from build123d import *

# Parameters (mm, degrees)
SKETCH1_W           = 80
SKETCH1_H           = 68
BOSS_EXTRUDE1_DEPTH = 45
CUT_EXTRUDE1_START  = 45
SKETCH2_W           = 76
SKETCH2_H           = 64
CUT_EXTRUDE1_DEPTH  = 33
SKETCH6_R           = 10.5
CUT_EXTRUDE10_DEPTH = 5
SKETCH7_W           = 30
SKETCH7_H           = 30
SKETCH7_W_2         = 26
SKETCH7_H_2         = 26
CUT_EXTRUDE11_DEPTH = 2
SKETCH8_R           = 1.5
CUT_EXTRUDE12_DEPTH = 3
SKETCH5_R           = 5.95
CUT_EXTRUDE14_DEPTH = 46
FILLET1_R           = 0.5
CUT_EXTRUDE15_START = 12
SKETCH12_R          = 24
CUT_EXTRUDE15_DEPTH = 5.5
BOSS_EXTRUDE5_START = -34
SKETCH13_W          = 80
SKETCH13_H          = 45
BOSS_EXTRUDE5_DEPTH = 16
CUT_EXTRUDE16_START = 45
SKETCH15_W          = 25
SKETCH15_H          = 16
CUT_EXTRUDE16_DEPTH = 33
SKETCH16_R          = 5.95
CUT_EXTRUDE17_DEPTH = 10
CUT_EXTRUDE18_START = 40
SKETCH17_R          = 5.6
CUT_EXTRUDE18_DEPTH = 50
CUT_EXTRUDE19_START = 40
SKETCH20_R          = 1
CUT_EXTRUDE19_DEPTH = 53
FILLET3_R           = 2
FILLET4_R           = 2
CUT_EXTRUDE20_START = 45
SKETCH21_W          = 51
SKETCH21_H          = 2
CUT_EXTRUDE20_DEPTH = 2
CUT_EXTRUDE22_START = 45
SKETCH22_W          = 2
SKETCH22_H          = 14
CUT_EXTRUDE22_DEPTH = 2
CUT_EXTRUDE23_START = -40
CUT_EXTRUDE23_DEPTH = 2


with BuildPart() as part:
    # Sketch1 → Boss-Extrude1 (new body)
    with BuildSketch(Plane(origin=(0, 0, 0), x_dir=(1, 0, 0), z_dir=(0, 1, 0))):
        Rectangle(SKETCH1_W, SKETCH1_H)
    extrude(amount=BOSS_EXTRUDE1_DEPTH)

    # Sketch2 → Cut-Extrude1 (cut)
    with BuildSketch(Plane(origin=(0, 0, 0), x_dir=(1, 0, 0), z_dir=(0, 1, 0)).offset(CUT_EXTRUDE1_START)):
        Rectangle(SKETCH2_W, SKETCH2_H)
    extrude(amount=-CUT_EXTRUDE1_DEPTH, mode=Mode.SUBTRACT)

    # Sketch6 → Cut-Extrude10 (cut)
    with BuildSketch(Plane.XZ):
        Circle(SKETCH6_R)
    extrude(amount=-CUT_EXTRUDE10_DEPTH, mode=Mode.SUBTRACT)

    # Sketch7 → Cut-Extrude11 (cut)
    with BuildSketch(Plane(origin=(0, 0, 0), x_dir=(-1, 0, 0), z_dir=(0, -1, 0))):
        Rectangle(SKETCH7_W, SKETCH7_H)
        Rectangle(SKETCH7_W_2, SKETCH7_H_2, mode=Mode.SUBTRACT)
    extrude(amount=-CUT_EXTRUDE11_DEPTH, mode=Mode.SUBTRACT)

    # Sketch8 → Cut-Extrude12 (cut, through all)
    with BuildSketch(Plane.ZY.offset(-38)):
        with Locations((29, 17)):
            Circle(SKETCH8_R)
    extrude(amount=-CUT_EXTRUDE12_DEPTH, mode=Mode.SUBTRACT)

    # Sketch5 → Cut-Extrude14 (cut, through all)
    with BuildSketch(Plane(origin=(0, 0, 0), x_dir=(1, 0, 0), z_dir=(0, 1, 0))):
        Circle(SKETCH5_R)
    extrude(amount=CUT_EXTRUDE14_DEPTH, mode=Mode.SUBTRACT)

    # Fillet1
    fillet1_edges = [part.edges().sort_by_distance(p)[0] for p in [
        (15, 0, 0),
        (0, 0, 15),
        (-15, 0, 0),
        (0, 0, -15),
        (13, 0, 0),
        (0, 0, -13),
        (-13, 0, 0),
        (0, 0, 13),
    ]]
    fillet(fillet1_edges, radius=FILLET1_R)

    # Sketch12 → Cut-Extrude15 (cut)
    with BuildSketch(Plane(origin=(0, 0, 0), x_dir=(1, 0, 0), z_dir=(0, 1, 0)).offset(CUT_EXTRUDE15_START)):
        Circle(SKETCH12_R)
    extrude(amount=-CUT_EXTRUDE15_DEPTH, mode=Mode.SUBTRACT)

    # Sketch13 → Boss-Extrude5 (add)
    with BuildSketch(Plane.XY.offset(BOSS_EXTRUDE5_START)):
        with Locations((0, 22.5)):
            Rectangle(SKETCH13_W, SKETCH13_H)
    extrude(amount=-BOSS_EXTRUDE5_DEPTH)

    # Sketch15 → Cut-Extrude16 (cut)
    with BuildSketch(Plane(origin=(0, 0, 0), x_dir=(1, 0, 0), z_dir=(0, 1, 0)).offset(CUT_EXTRUDE16_START)):
        with Locations((-25.5, 40)):
            Rectangle(SKETCH15_W, SKETCH15_H)
    extrude(amount=-CUT_EXTRUDE16_DEPTH, mode=Mode.SUBTRACT)

    # Sketch16 → Cut-Extrude17 (cut)
    with BuildSketch(Plane(origin=(0, 12, 0), x_dir=(1, 0, 0), z_dir=(0, 1, 0))):
        with Locations((-25.5, 40)):
            Circle(SKETCH16_R)
    extrude(amount=-CUT_EXTRUDE17_DEPTH, mode=Mode.SUBTRACT)

    # Sketch17 → Cut-Extrude18 (cut)
    with BuildSketch(Plane(origin=(0, 0, 0), x_dir=(0, 0, -1), z_dir=(1, 0, 0)).offset(CUT_EXTRUDE18_START)):
        with Locations((39.6, 20.00233054)):
            Circle(SKETCH17_R)
    extrude(amount=-CUT_EXTRUDE18_DEPTH, mode=Mode.SUBTRACT)

    # Sketch20 → Cut-Extrude19 (cut)
    with BuildSketch(Plane(origin=(0, 0, 0), x_dir=(0, 0, -1), z_dir=(1, 0, 0)).offset(CUT_EXTRUDE19_START)):
        with Locations((44.775, 25.17733054)):
            Circle(SKETCH20_R)
        with Locations((34.425, 14.82733054)):
            Circle(SKETCH20_R)
    extrude(amount=-CUT_EXTRUDE19_DEPTH, mode=Mode.SUBTRACT)

    # Fillet3
    fillet3_edges = [part.edges().sort_by_distance(p)[0] for p in [
        (-40, 22.5, -50),
        (40, 22.5, 34),
        (-40, 22.5, 34),
        (40, 22.5, -50),
    ]]
    fillet(fillet3_edges, radius=FILLET3_R)

    # Fillet4
    fillet4_edges = [part.edges().sort_by_distance(p)[0] for p in [
        (40, 0, -8),
        (0, 0, 34),
        (-40, 0, -8),
        (0, 0, -50),
        (-39.414213562, 0, 33.414213562),
        (-39.414213562, 0, -49.414213562),
        (39.414213562, 0, -49.414213562),
        (39.414213562, 0, 33.414213562),
    ]]
    fillet(fillet4_edges, radius=FILLET4_R)

    # Sketch21 → Cut-Extrude20 (cut)
    with BuildSketch(Plane(origin=(0, 0, 0), x_dir=(1, 0, 0), z_dir=(0, 1, 0)).offset(CUT_EXTRUDE20_START)):
        with Locations((12.5, 47)):
            Rectangle(SKETCH21_W, SKETCH21_H)
    extrude(amount=-CUT_EXTRUDE20_DEPTH, mode=Mode.SUBTRACT)

    # Sketch22 → Cut-Extrude22 (cut)
    with BuildSketch(Plane(origin=(0, 0, 0), x_dir=(1, 0, 0), z_dir=(0, 1, 0)).offset(CUT_EXTRUDE22_START)):
        with Locations((37, 39)):
            Rectangle(SKETCH22_W, SKETCH22_H)
    extrude(amount=-CUT_EXTRUDE22_DEPTH, mode=Mode.SUBTRACT)

    # Sketch23 → Cut-Extrude23 (cut)
    with BuildSketch(Plane(origin=(0, 0, 0), x_dir=(0, 0, -1), z_dir=(1, 0, 0)).offset(CUT_EXTRUDE23_START)):
        with BuildLine():
            Line((-20.205872853, 31), (24.794127147, 31))
            ThreePointArc((24.794127147, 31), (25.794127147, 30), (24.794127147, 29))
            Line((24.794127147, 29), (-20.205872853, 29))
            ThreePointArc((-20.205872853, 29), (-21.205872853, 30), (-20.205872853, 31))
        make_face()
    extrude(amount=CUT_EXTRUDE23_DEPTH, mode=Mode.SUBTRACT)


solid = part.part
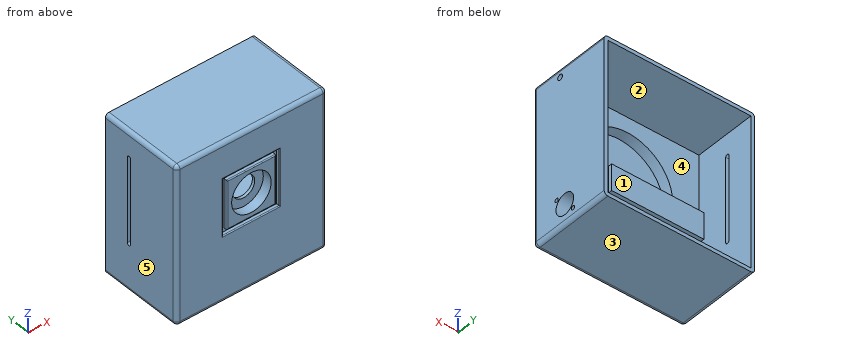
Verification items for the finished model (mm, model axes). Face numbers are marked on the shaded views. A direction names the side the tool comes from. Give positions to 0.01 mm unless a question says otherwise; leave off trailing zeros. Write each loop counter-clockwise with the first axis right and the second up, starting at its lowest first coordinate (ties: lowest second). Pieces come first, ordered by that corner, then holes. Notation, with made-up numbers: (84, 61) - (92, 61) arc R15 cw to (92, 65) - close; hole circle Ø6 at (42, -34.5). An arc over 180 degrees is marked (long way). Answer as CSV lines item,"result". Start each with the question number.
1. Draft check along X on the marked faces 3, 4 and 5. Enter one of: pulls with the +X half, pulls with the -X half, needs draft (parallel to the pull), parting line crosses it, or undercut.
2. Sectioned sample at A-A (z = 29). Record the boundary of the cut face in (x, y).
3. Thickness scan on line 1 (X direction, y = 39, z = -39.5); line 2 (Z direction, x = 0, y = 10.05); line 3 (X direction, y = 25, z = 12). Record the ranges inside material, lowest first.
4. Sectioned sample at C-C (y = 4). Record the boundary of the cut face in (x, z), then the cut area to 3 significant figures.
5. Sectioned sample at D-D (x = 0). Count the separate pieces of the cut face and the enclosed holes in it, then the cut area to 3 significant figures.
6. Sectioned sample at B-B (x = -25.5). Record the boundary of the cut face in (y, z), then the cut area to 3 significant figures.
7. Set-up check for the marked faces 1 and 2: record each of +Z, -Z, +X, -X, +Y, -Y from which the full face is reachable in a straight line by a thin tool's end or side.
8. Depth check by flat-ended pin: pin 1 (12 mm diameter, centred on x = -12.5, z = -14, fed in from +Y); pin 2 (10.5 mm diameter, centred on x = 0, z = 0, fed in from -Y); pin 3 (1.6 mm diameter, centred on y = 1, z = -4, fed in from +X); pin 4 (0.8 mm diameter, centred on x = 6.5, y = 1, fed in from +Z). Enter the tip coordinate at first touch or a pass-through.
Derived:
1,face 3,"needs draft"
1,face 4,"undercut"
1,face 5,"pulls with the -X half"
2,outline,"(-40, 2) arc R2 ccw to (-38, 0) - (38, 0) arc R2 ccw to (40, 2) - (40, 15.5) - (38, 15.5) - (38, 12) - (-38, 12) - (-38, 45) - (-40, 45) - close; (38, 18.5) - (40, 18.5) - (40, 45) - (38, 45) - close"
3,line 1,"-40 to -38, -13 to 40"
3,line 2,"-50 to -24, 24 to 34"
3,line 3,"-40 to -38, 38 to 40"
4,outline,"(-40, -48) arc R2 ccw to (-38, -50) - (38, -50) arc R2 ccw to (40, -48) - (40, 32) arc R2 ccw to (38, 34) - (-38, 34) arc R2 ccw to (-40, 32) - close; hole circle Ø11.9 at (-25.5, -40); hole circle Ø21 at (0, 0)"
4,area,"6,260 mm²"
5,separate pieces,"2"
5,enclosed holes,"3"
5,area,"1,160 mm²"
6,outline,"(0, -48) arc R2 ccw to (2, -50) - (45, -50) - (45, -48) - (12, -48) - (12, -45.95) - (2, -45.95) - (2, -34.05) - (12, -34.05) - (12, 32) - (45, 32) - (45, 34) - (2, 34) arc R2 ccw to (0, 32) - close"
6,area,"1,020 mm²"
7,face 1,"+Z, -Z, +X, -X, +Y"
7,face 2,"+Y"
8,pin 1,"y = 12"
8,pin 2,"through"
8,pin 3,"x = 39.99"
8,pin 4,"z = 33.91"
